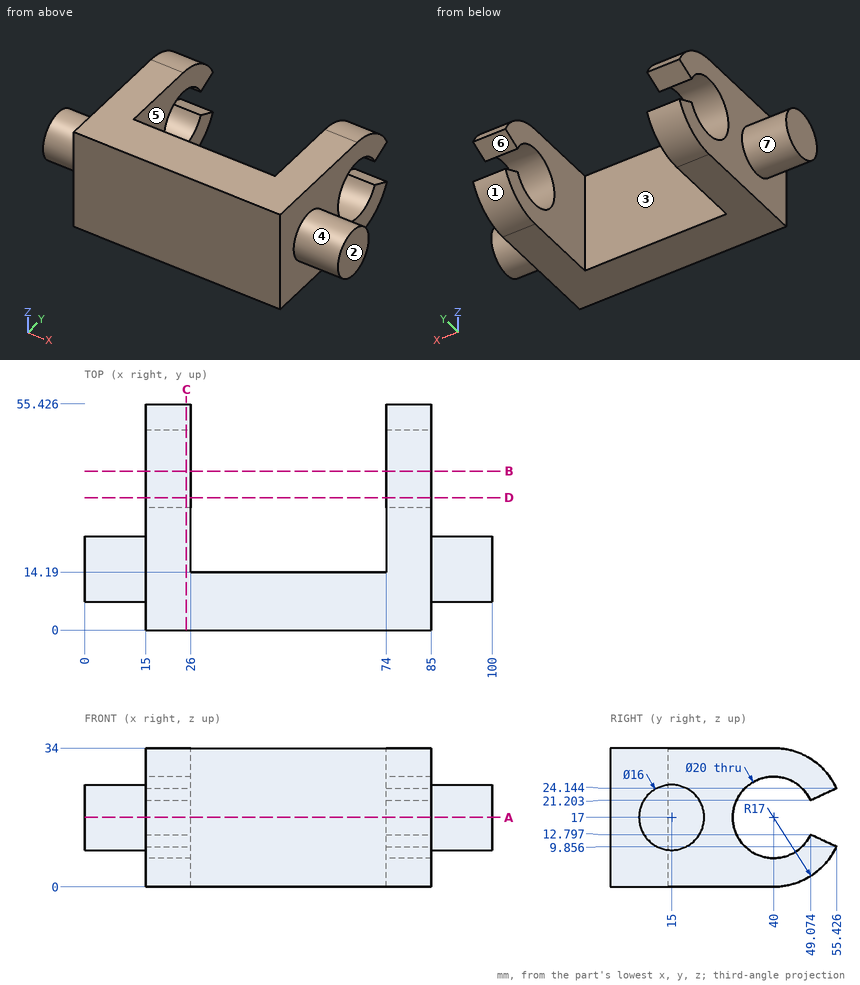
Check sheet for the drawn part. Datum: minimum x, y, z corner. Units: mm. A direction names the side the tool comes from. Coordinates: 2 decimals unless noted, no trailing zeros. Write each loop counter-clockwise with the first axis right and the second up, starting at its lowest first coordinate (ties: lowest second). Pieces come first, ordered by that corner, then holes. Notation, with made-up numbers: M 74.25,-4 L 131.25,-4 A18 cw 131.25,31 Z; hole C -22.5,49 d8. An arc over 180 degrees is marked long. One line per item, written item: value.
Item 1: Section check D-D, the plane y = 32.5. Record the boundary of the cut face in (x, z) (1 decimal), plus the area to 3 significant figures.
Check sheet entries:
outline: M 15,0 L 26,0 L 26,10.4 L 15,10.4 Z; M 15,23.6 L 26,23.6 L 26,34 L 15,34 Z; M 74,0 L 85,0 L 85,10.4 L 74,10.4 Z; M 74,23.6 L 85,23.6 L 85,34 L 74,34 Z
area: 457 mm^2
Item 2: Scan lines: line 1 along Z through (x, y) = (23, 40); line 2 along X through (y, z) = (40, 32); line 3 along X through (y, z) = (18, 21.5). Record each from-to range of solid material in increasing order.
Check sheet entries:
line 1: z = 0 to 7, 27 to 34
line 2: x = 15 to 26, 74 to 85
line 3: x = 0 to 26, 74 to 100
Item 3: Access from +Z, -Z, +X, -X, +Y, -Y to the whole of each face (thin tool, end or side, straight path). Record for the marked faces 4, 5, 6 and 7.
Check sheet entries:
face 4: +X
face 5: +Z, -Z, +Y
face 6: +X, -X, +Y
face 7: -X
Item 4: Gauge pin test, flat end, axial feed: pin 1 Ø1 at (y, z) = (49.5, 10.5) entering from -X. Record the tip position at first contact, or that the pin passes through.
Check sheet entries:
pin 1: stops at x = 15
Item 5: Mould release check, pull along X, two halves, no side actions. Record for the marked faces 1, 2 and 3: pulls with the +X half, pulls with the -X half, needs draft (parallel to the pull), parting line crosses it, or undercut.
Check sheet entries:
face 1: needs draft
face 2: pulls with the +X half
face 3: undercut
Item 6: Section check B-B, the plane y = 39. Record the boundary of the cut face in (x, z).
Check sheet entries:
outline: M 15,0 L 26,0 L 26,7.05 L 15,7.05 Z; M 15,26.95 L 26,26.95 L 26,34 L 15,34 Z; M 74,0 L 85,0 L 85,7.05 L 74,7.05 Z; M 74,26.95 L 85,26.95 L 85,34 L 74,34 Z
Item 7: Section check C-C, the plane x = 25. Record the boundary of the cut face in (y, z) (1 decimal).
Check sheet entries:
outline: M 0,0 L 40,0 A17 ccw 55.4,9.9 L 49.1,12.8 A10 cw long 49.1,21.2 L 55.4,24.1 A17 ccw 40,34 L 0,34 Z
Item 8: Section check A-A, the plane z = 17. Record the boundary of the cut face in (x, y).
Check sheet entries:
outline: M 0,7 L 15,7 L 15,0 L 85,0 L 85,7 L 100,7 L 100,23 L 85,23 L 85,30 L 74,30 L 74,14.19 L 26,14.19 L 26,30 L 15,30 L 15,23 L 0,23 Z
